Geometry check sheet. Reference: the model listing, model coordinates, mm. Round coordinates to 2 decimals unless told otherwise and drop trailing zeros. Write each loop counter-clockwise with the first axis right and the second up, starting at its lowest first coordinate (ties: lowest second). Pieces come first, ordered by that corner, then holes. Notation, with made-up numbers: (-21.75, -15) -> (6.25, -15) arc R10 ccw to (6.25, 2) -> close; hole circle Ø6 at (51.25, 33.25). An arc over 180 degrees is marked (long way). Put each result on its own line as item: value. Start each with the question number.
from build123d import *

# Parameters (mm, degrees)
F0_W     = 101.6
F0_H     = 76.2
F1_DEPTH = 9.525
F2_R     = 3.4925
F3_DEPTH = 25.4
F4_R     = 3.4925
F5_DEPTH = 25.4
F6_R     = 1.5875
F7_DEPTH = 25.4
F9_D     = 5.1054
F9_DEPTH = 12.7
F9_TIP   = 1.5338169022


with BuildPart() as f1:
    # F0 (on Front) → F1 (new body, symmetric)
    with BuildSketch(Plane.XZ):
        with Locations((-12.7, 0)):
            Rectangle(F0_W, F0_H)
    extrude(amount=F1_DEPTH, both=True)

    # F2 (on face) → F3 (cut)
    with BuildSketch(Plane.XZ.offset(9.525)):
        with Locations((11.8585942021, 28.6291789535)):
            Circle(F2_R)
        with Locations((-11.8585942021, 28.6291789535)):
            Circle(F2_R)
        with Locations((-28.6291789535, 11.8585942021)):
            Circle(F2_R)
        with Locations((-28.6291789535, -11.8585942021)):
            Circle(F2_R)
        with Locations((-11.8585942021, -28.6291789535)):
            Circle(F2_R)
        with Locations((11.8585942021, -28.6291789535)):
            Circle(F2_R)
        with Locations((28.6291789535, -11.8585942021)):
            Circle(F2_R)
        with Locations((28.6291789535, 11.8585942021)):
            Circle(F2_R)
    extrude(amount=-F3_DEPTH, mode=Mode.SUBTRACT)

    # F4 (on face) → F5 (cut)
    with BuildSketch(Plane.XZ.offset(9.525)):
        with Locations((-50.8, 0)):
            Circle(F4_R)
    extrude(amount=-F5_DEPTH, mode=Mode.SUBTRACT)

    # F6 (on face) → F7 (cut)
    with BuildSketch(Plane.XZ.offset(9.525)):
        with Locations((17.4625, 0)):
            Circle(F6_R)
    extrude(amount=-F7_DEPTH, mode=Mode.SUBTRACT)

    # F9
    with Locations(Plane.XZ.offset(9.525)):
        with Locations((17.4625, 0)):
            Hole(F9_D / 2, depth=F9_DEPTH)
            with Locations((0, 0, -(F9_DEPTH + F9_TIP / 2))):  # 118° drill point
                Cone(0, F9_D / 2, F9_TIP, mode=Mode.SUBTRACT)


solid = f1.part
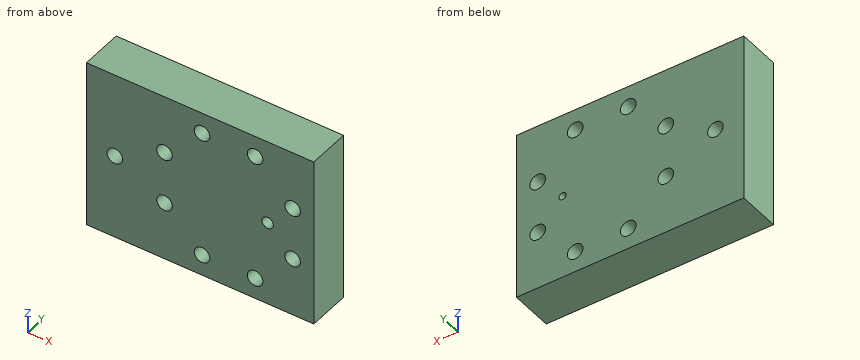
(1) Sectioned sample at D-D (z = 10). Record the cut outline in (x, y) (3 decimals), and give its area (3 significant figures).
(2) Sectioned sample at B-B (x = -50.8). Record the cut outline in (y, z) (1 decimal).
(3) Go/stop test with flat-tipped pins: pin 1 Ø4 at (x, z) = (17.46, 0) entering from -Y; pin 2 Ø9 at (x, z) = (-11.86, 28.63) entering from -Y (3 decimals); pin 3 Ø4 at (x, z) = (-28.63, -11.86) entering from -Y. Record where each tip stops, or that it passes through.
(4) Sectioned sample at A-A (z = 0). State how many separate pieces and enclosed holes the cut face has, and give its area (3 significant figures).
(5) Material ranges on L1, parallel to Z at x = 12, y = 3; L2, parallel to Z at x = 29, y = -2; L3, parallel to Z at x = -50.8, y = 2, recorded low to high. Write a range as from..to.
Found:
1. outline: (-63.5, -9.525) -> (-31.586, -9.525) -> (-31.586, 9.525) -> (-63.5, 9.525) -> close; (-25.672, -9.525) -> (25.672, -9.525) -> (25.672, 9.525) -> (-25.672, 9.525) -> close; (31.586, -9.525) -> (38.1, -9.525) -> (38.1, 9.525) -> (31.586, 9.525) -> close
1. area: 1,710 mm2
2. outline: (-9.5, -38.1) -> (9.5, -38.1) -> (9.5, -3.5) -> (-9.5, -3.5) -> close; (-9.5, 3.5) -> (9.5, 3.5) -> (9.5, 38.1) -> (-9.5, 38.1) -> close
3. pin 1: y = 3.51
3. pin 2: y = -9.525
3. pin 3: through
4. separate pieces: 3
4. enclosed holes: 0
4. area: 1,720 mm2
5. L1: -38.1..-32.12, -25.14..25.14, 32.12..38.1
5. L2: -38.1..-15.33, -8.39..8.39, 15.33..38.1
5. L3: -38.1..-3.49, 3.49..38.1
